The figure shows three views and two pictorial views of one solid part (mm, origin at its lowest corner). Answer the questions. A direction names the side the tool comes from. Give positions to 0.01 mm unless a question says otherwise; leave off trailing zeros. Write each loop counter-clockwise with the first axis right and the second up, starting at its lowest first coordinate (ties: lowest second). Pieces come first, ordered by that corner, then holes. Notation, with made-up numbers: (9.5, -38) -> (31.5, -38) arc R23 cw to (31.5, -29) -> close; hole circle Ø9 at (65, 78.5). An arc over 180 degrees is marked (long way). Write item = value, one per line. Start each with the question number.
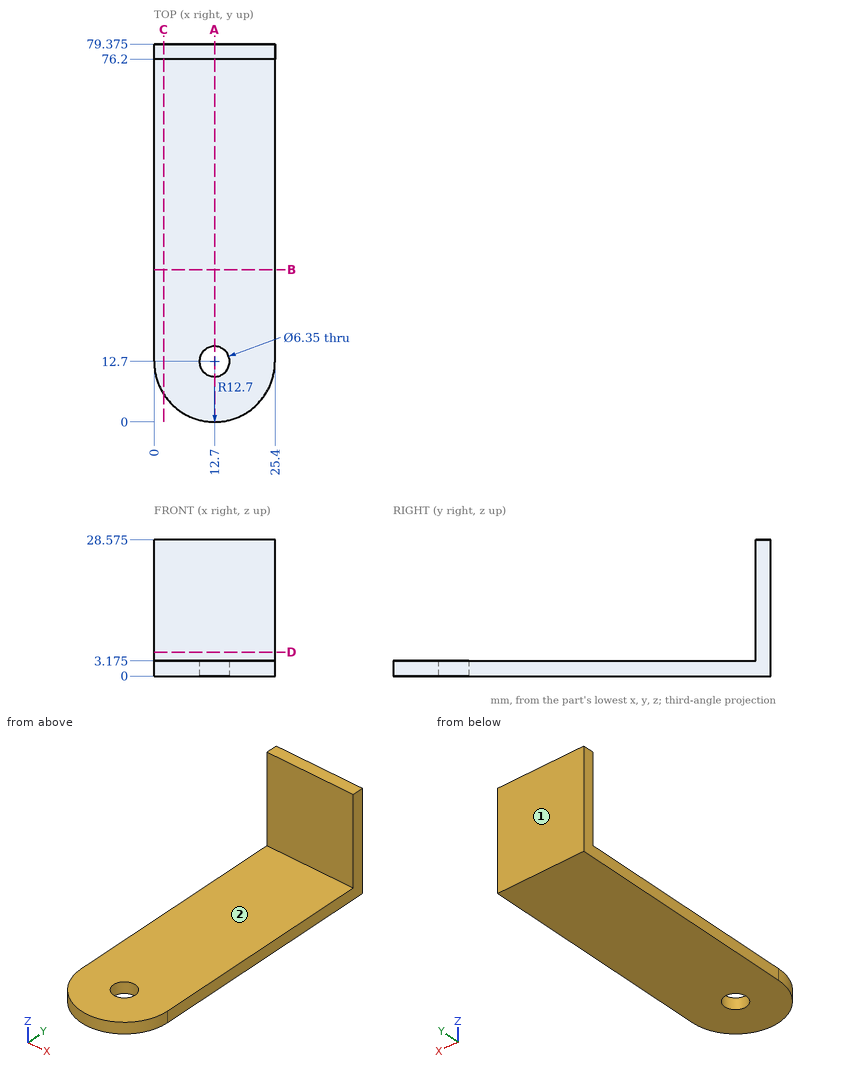
(1) A cutting plane is placed at B-B, the plane y = 32. Write down the section's boundary in (x, z) (3 decimals).
(2) A cutting plane is placed at C-C, the plane x = 2. Write down the section's boundary in (y, z) (3 decimals), then the cut area to 3 significant figures.
(3) Each of these flat-tipped pins is pushed along its axis until it touches: pin 1 (1 mm diameter, centred on x = 20.5, z = 4.5, fed in from -Y); pin 2 (1.5 mm diameter, centred on x = 4, y = 68, fed in from +Z) (3 decimals); pin 3 (5 mm diameter, centred on y = 30.5, z = 7.5, fed in from +X). Where does it stop, or does it pass through?
(4) A cutting plane is placed at D-D, the plane z = 5. Write down the section's boundary in (x, y) (3 decimals), then the cut area to 3 significant figures.
(5) Find the intervals of material crossed by line 1 along Y through (x, z) = (12.7, 2.45) (3 decimals); line 2 along Y through (x, z) = (1.25, 17.5) (3 decimals); line 3 along Z through (x, y) = (8, 3) (3 decimals), in increasing order.
(6) A cutting plane is placed at A-A, the plane x = 12.7. Write down the section's boundary in (y, z) (3 decimals), then the cut area to 4 significant figures.
(7) For the marked faces 1 and 2, determine the directions among +Z, -Z, +X, -X, +Y, -Y from which every point of the face is accessible in a straight line to the end or side of a thin tool.
Results list:
q1.outline = (0, 0) -> (25.4, 0) -> (25.4, 3.175) -> (0, 3.175) -> close
q2.outline = (5.859, 0) -> (79.375, 0) -> (79.375, 28.575) -> (76.2, 28.575) -> (76.2, 3.175) -> (5.859, 3.175) -> close
q2.area = 314 mm²
q3.pin_1 = 76.2
q3.pin_2 = 3.175
q3.pin_3 = through
q4.outline = (0, 76.2) -> (25.4, 76.2) -> (25.4, 79.375) -> (0, 79.375) -> close
q4.area = 80.6 mm²
q5.line_1 = 0 to 9.525, 15.875 to 79.375
q5.line_2 = 76.2 to 79.375
q5.line_3 = 0 to 3.175
q6.outline = (0, 0) -> (9.525, 0) -> (9.525, 3.175) -> (0, 3.175) -> close; (15.875, 0) -> (79.375, 0) -> (79.375, 28.575) -> (76.2, 28.575) -> (76.2, 3.175) -> (15.875, 3.175) -> close
q6.area = 312.5 mm²
q7.face_1 = +Z, -Z, +X, -X, +Y
q7.face_2 = +Z, +X, -X, -Y
